Could you check a few things on this drawing? It's one solid part, dimensions in mm from its lowest x, y, z. Give positions to 0.01 mm unless a question says otherwise; leave off trailing zeros. Loops run counter-clockwise (first coordinate to the right, second up) from the corner with the lowest first, then second, coordinate; pieces in that order, holes last. Notation, with made-up numbers: (-13, 45.25) - (32, 45.25) arc R16 ccw to (32, 66.25) - close; hole circle Ø11 at (48.25, 69). An arc over 180 degrees is marked (long way). Answer as a JSON object with one key per item and string values.
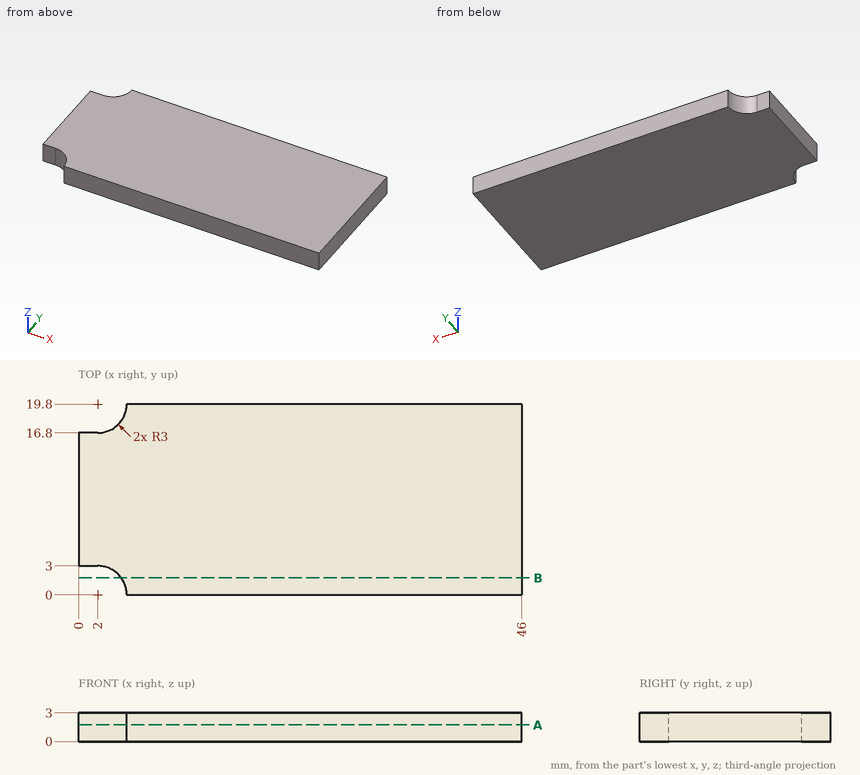
1) Imagine slicing it at B-B on y = 1.75. Write out the boundary of the cut face in (x, z).
Check sheet entries:
{"outline": "(4.44, 0) - (46, 0) - (46, 3) - (4.44, 3) - close"}
2) Imagine slicing it at A-A on z = 1.75. Write out the boundary of the cut face in (x, y), and give its area (3 significant figures).
Check sheet entries:
{"outline": "(0, 3) - (2, 3) arc R3 cw to (5, 0) - (46, 0) - (46, 19.8) - (5, 19.8) arc R3 cw to (2, 16.8) - (0, 16.8) - close", "area": "885 mm2"}
3) I need wall thicknesses on L1, parallel to X at y = 19.25, z = 1.75; L2, parallel to X at y = 18.5, z = 0.85; L3, parallel to Y at x = 4.5, z = 2.6. Which ranges of each line are inside material? Lowest first, please.
Check sheet entries:
{"L1": "4.95 to 46", "L2": "4.7 to 46", "L3": "1.66 to 18.14"}
4) I'm going to push a flat-ended pin straight in: P1, Ø1.5, axis at x = 37.5, y = 14, coming from the -Z side. Where does the tip first touch, or does it pass through?
Check sheet entries:
{"P1": "z = 0"}
